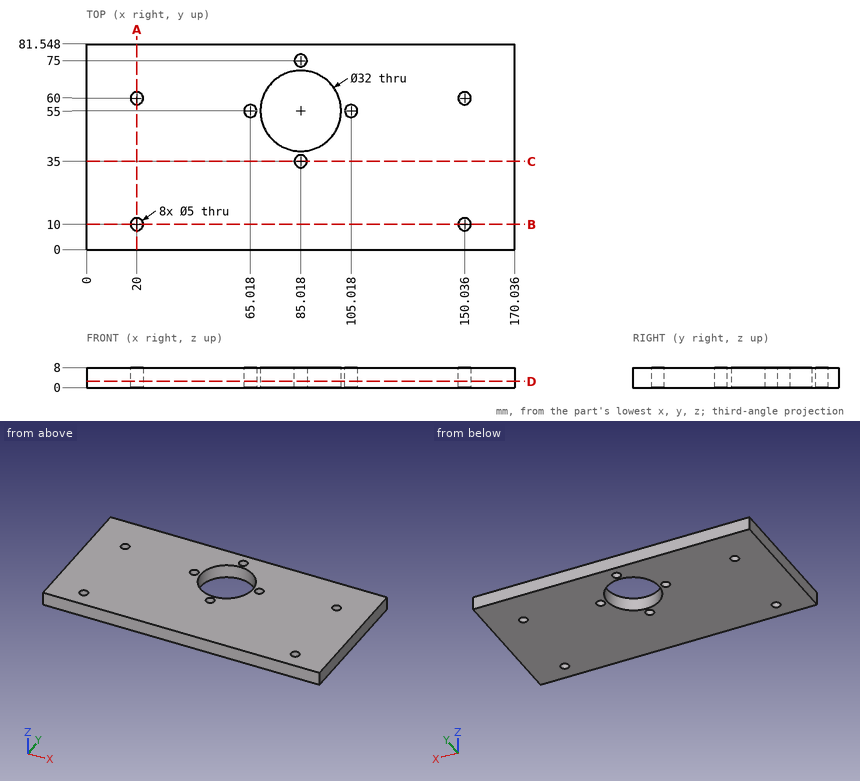
Study the drawing (mm; zero at the part's minimum x, y, z) and answer. Give positions to 0.01 mm unless a question says otherwise; leave off trailing zeros. Order: outer loops, then holes, each group sorted by start corner. A loop starts at its lowest first (then second) coordinate and runs counter-clockwise, first axis right, second up. Notation, with made-up numbers: (36.25, 44.25) - (89.25, 44.25) arc R24 ccw to (89.25, 59.25) - close; hole circle Ø8 at (-25.75, 24). An arc over 180 degrees is marked (long way). Answer as CSV lines item,"result". Start each with the question number.
Q1. The part is cut by section D-D (z = 2.5). Give the number of separate pieces and of enclosed holes in the cut face, then the cut area to 3 significant figures.
Q2. The part is cut by section A-A (x = 20). Write down the section's boundary in (y, z).
Q3. Given pin 1 Ø8 at (x, y) = (65.02, 55) entering from -Z; pin 2 Ø4.5 at (x, y) = (85.02, 35) entering from -Z, each flat-ended and moving along its own axis, determine where each tip first touches the part or whether it passes through.
Q4. The part is cut by section C-C (y = 35). Write down the section's boundary in (x, z) (1 decimal), then the cut area to 3 significant figures.
Q5. Find the intervals of material crossed by L1, parallel to Y at x = 20, z = 6; L2, parallel to Y at x = 86, z = 4; L3, parallel to Y at x = 149, z = 5.25 (1 decimal), in increasing order. Write a range as [from, to].
Q6. The part is cut by section B-B (y = 10). Write down the section's boundary in (x, z) (1 decimal).
Check result:
1,separate pieces,"1"
1,enclosed holes,"9"
1,area,"12,900 mm²"
2,outline,"(0, 0) - (7.5, 0) - (7.5, 8) - (0, 8) - close; (12.5, 0) - (57.5, 0) - (57.5, 8) - (12.5, 8) - close; (62.5, 0) - (81.55, 0) - (81.55, 8) - (62.5, 8) - close"
3,pin 1,"stops at z = 0"
3,pin 2,"passes through"
4,outline,"(0, 0) - (82.5, 0) - (82.5, 8) - (0, 8) - close; (87.5, 0) - (170, 0) - (170, 8) - (87.5, 8) - close"
4,area,"1,320 mm²"
5,L1,"y = [0, 7.5], [12.5, 57.5], [62.5, 81.55]"
5,L2,"y = [0, 32.7], [37.3, 39.03], [70.97, 72.7], [77.3, 81.55]"
5,L3,"y = [0, 7.7], [12.3, 57.7], [62.3, 81.5]"
6,outline,"(0, 0) - (17.5, 0) - (17.5, 8) - (0, 8) - close; (22.5, 0) - (147.5, 0) - (147.5, 8) - (22.5, 8) - close; (152.5, 0) - (170, 0) - (170, 8) - (152.5, 8) - close"
